from build123d import *

# Parameters (mm, degrees)
SKETCH1_R           = 3
BOSS_EXTRUDE1_DEPTH = 1
CHAMFER1_SIZE       = 1


with BuildPart() as part:
    # Sketch1 → Boss-Extrude1 (new body)
    with BuildSketch(Plane(origin=(0, 0, 0), x_dir=(1, 0, 0), z_dir=(0, 1, 0))):
        with BuildLine():
            Line((-500, -1000), (500, -1000))
            Line((500, -1000), (500, -100))
            ThreePointArc((500, -100), (400, 0), (500, 100))
            Line((500, 100), (500, 1000))
            Line((500, 1000), (-500, 1000))
            Line((-500, 1000), (-500, -1000))
        make_face()
        with Locations(Location((-480, 490, 0), (0, 0, 270))):
            Circle(SKETCH1_R, mode=Mode.SUBTRACT)
        with Locations(Location((-480, -980, 0), (0, 0, 270))):
            Circle(SKETCH1_R, mode=Mode.SUBTRACT)
        with Locations(Location((480, -980, 0), (0, 0, 270))):
            Circle(SKETCH1_R, mode=Mode.SUBTRACT)
        with Locations(Location((480, 980, 0), (0, 0, 270))):
            Circle(SKETCH1_R, mode=Mode.SUBTRACT)
        with Locations(Location((-480, 980, 0), (0, 0, 270))):
            Circle(SKETCH1_R, mode=Mode.SUBTRACT)
        with Locations(Location((-480, 0, 0), (0, 0, 270))):
            Circle(SKETCH1_R, mode=Mode.SUBTRACT)
        with Locations(Location((-480, -490, 0), (0, 0, 270))):
            Circle(SKETCH1_R, mode=Mode.SUBTRACT)
        with Locations(Location((0, -980, 0), (0, 0, 270))):
            Circle(SKETCH1_R, mode=Mode.SUBTRACT)
        with Locations(Location((0, 980, 0), (0, 0, 270))):
            Circle(SKETCH1_R, mode=Mode.SUBTRACT)
    extrude(amount=BOSS_EXTRUDE1_DEPTH)

    # Chamfer1
    chamfer1_edges = [part.edges().sort_by_distance(p)[0] for p in [
        (0, 1, -983),
        (0, 1, 977),
        (-480, 1, 487),
        (-480, 1, -3),
        (-480, 1, -983),
        (480, 1, -983),
        (480, 1, 977),
        (-480, 1, 977),
        (-480, 1, -493),
    ]]
    chamfer(chamfer1_edges, length=CHAMFER1_SIZE - 0.0001)  # a hair under: the kernel refuses the full size


solid = part.part
CAD build for the part. Positions are in the model's coordinates, mm. Round coordinates to 2 decimals unless told otherwise and drop trailing zeros. Write each loop counter-clockwise with the first axis right and the second up, starting at its lowest first coordinate (ties: lowest second). Pieces come first, ordered by that corner, then holes.
(1) Probe line 1 along Z through (x, y) = (1, 0.3); line 2 along X through (y, z) = (0.05, 980); line 3 along Z through (x, y) = (-480, 0.05). List the from-to ranges inside material, lowest first.
(2) Mould opens along Z. For faces 1 (the face through (400.024, 0.493, 2.199)), 2 (the face through (-7, 0, -14)) say: pulls with the +Z half, pulls with the -Z half, needs draft (parallel to the pull), parting line crosses it, or undercut.
(3) Drop flat-ended pins along their axis: P1, Ø5.5, axis at x = -480, z = 0, coming from the +Y side; P2, Ø7, axis at x = -480, z = 490, coming from the +Y side. Give the stop position or say it passes through.
(4) Slice it at A-A, the plane z = 55. Write the cut outline in (x, y), and give its area (3 significant figures).
From the geometry:
1. line 1: z = -1000 to -983.14, -976.86 to 976.86, 983.14 to 1000
1. line 2: x = -500 to -483.05, -476.95 to -3.05, 3.05 to 476.95, 483.05 to 500
1. line 3: z = -1000 to -983.05, -976.95 to -493.05, -486.95 to -3.05, 3.05 to 486.95, 493.05 to 976.95, 983.05 to 1000
2. face 1: undercut
2. face 2: needs draft
3. P1: passes through
3. P2: stops at y = 0.5
4. outline: (-500, 0) - (416.48, 0) - (416.48, 1) - (-500, 1) - close
4. area: 916 mm2
